from build123d import *

# Parameters (mm, degrees)
SKETCH_1_R      = 1.5
SKETCH_1_R_2    = 2
SKETCH_1_R_3    = 6.2
EXTRUDE_1_DEPTH = 3


with BuildPart() as part:
    # 草图1 → 凸台-拉伸1 (new body)
    with BuildSketch(Plane.XY):
        with BuildLine():
            Line((2522.174251857, 1992.03397428), (2522.174251857, 1983.327521496))
            Line((2522.174251857, 1983.327521496), (2519.174251857, 1983.327521496))
            Line((2519.174251857, 1983.327521496), (2519.174251857, 1975.827521496))
            Line((2519.174251857, 1975.827521496), (2522.174251857, 1975.827521496))
            Line((2522.174251857, 1975.827521496), (2522.174251857, 1965.121068713))
            Line((2522.174251857, 1965.121068713), (2517.424251857, 1965.121068713))
            Line((2517.424251857, 1965.121068713), (2517.424251857, 1968.121068713))
            Line((2517.424251857, 1968.121068713), (2509.924251857, 1968.121068713))
            Line((2509.924251857, 1968.121068713), (2509.924251857, 1965.121068713))
            Line((2509.924251857, 1965.121068713), (2498.924251857, 1965.121068713))
            Line((2498.924251857, 1965.121068713), (2498.924251857, 1968.121068713))
            Line((2498.924251857, 1968.121068713), (2491.424251857, 1968.121068713))
            Line((2491.424251857, 1968.121068713), (2491.424251857, 1965.121068713))
            Line((2491.424251857, 1965.121068713), (2480.424251857, 1965.121068713))
            Line((2480.424251857, 1965.121068713), (2480.424251857, 1968.121068713))
            Line((2480.424251857, 1968.121068713), (2472.924251857, 1968.121068713))
            Line((2472.924251857, 1968.121068713), (2472.924251857, 1965.121068713))
            Line((2472.924251857, 1965.121068713), (2468.174251857, 1965.121068713))
            Line((2468.174251857, 1965.121068713), (2468.174251857, 1975.827521496))
            Line((2468.174251857, 1975.827521496), (2471.174251857, 1975.827521496))
            Line((2471.174251857, 1975.827521496), (2471.174251857, 1983.327521496))
            Line((2471.174251857, 1983.327521496), (2468.174251857, 1983.327521496))
            Line((2468.174251857, 1983.327521496), (2468.174251857, 1992.03397428))
            ThreePointArc((2468.174251857, 1992.03397428), (2495.174251857, 2019.03397428), (2522.174251857, 1992.03397428))
        make_face()
        with Locations((2472.663889086, 1992.03397428)):
            Circle(SKETCH_1_R, mode=Mode.SUBTRACT)
        with Locations((2483.919070472, 2011.528520288)):
            Circle(SKETCH_1_R, mode=Mode.SUBTRACT)
        with Locations((2506.429433243, 2011.528520288)):
            Circle(SKETCH_1_R, mode=Mode.SUBTRACT)
        with Locations((2517.684614628, 1992.03397428)):
            Circle(SKETCH_1_R, mode=Mode.SUBTRACT)
        with Locations((2501.338054428, 1969.0074786)):
            Circle(SKETCH_1_R_2, mode=Mode.SUBTRACT)
        with Locations((2483.919070472, 1972.539428272)):
            Circle(SKETCH_1_R, mode=Mode.SUBTRACT)
        with Locations((2506.429433243, 1972.539428272)):
            Circle(SKETCH_1_R, mode=Mode.SUBTRACT)
        with Locations((2489.010449286, 1969.0074786)):
            Circle(SKETCH_1_R_2, mode=Mode.SUBTRACT)
        with Locations((2495.174251857, 1992.03397428)):
            Circle(SKETCH_1_R_3, mode=Mode.SUBTRACT)
    extrude(amount=EXTRUDE_1_DEPTH)


solid = part.part
Part model, mm, in its own coordinate system. A direction names the side the tool comes from. Give positions to 0.01 mm unless a question says otherwise; leave off trailing zeros. Write each loop counter-clockwise with the first axis right and the second up, starting at its lowest first coordinate (ties: lowest second). Pieces come first, ordered by that corner, then holes.
1) Two-plate mould, pull along Y, no slides. Class faces 1 (the face through (2486, 1965.121, 1)), 2 (the face through (2500.9, 1989.66, 1.48)), 3 (the face through (2509.924, 1967, 1)): released by +Y, released by -Y, zero draft, split by the parting line, or undercut.
Resolved:
face 1: released by -Y
face 2: undercut
face 3: zero draft
2) Cut at A-A on y = 1989.5. Write the cut outline in (x, z).
Resolved:
outline: (2468.17, 0) - (2489.52, 0) - (2489.52, 3) - (2468.17, 3) - close; (2500.83, 0) - (2522.17, 0) - (2522.17, 3) - (2500.83, 3) - close
3) Cut at B-B on x = 2497. Write the cut outline in (y, z).
Resolved:
outline: (1968.12, 0) - (1986.11, 0) - (1986.11, 3) - (1968.12, 3) - close; (1997.96, 0) - (2018.97, 0) - (2018.97, 3) - (1997.96, 3) - close
4) Which spindle directions (+Z, -Z, +X, -X, +Y, -Y) get a long thin tool onto all of the face, cutting with end or side? Do faces 4 (the face through (2505, 1973, 1)), 5 (the face through (2495, 1968.121, 1)), 6 (the face through (2521, 1983.328, 1)), 7 (the face through (2471.174, 1980, 1)), 8 (the face through (2502, 1992, 3)). Say none if no direction does.
Resolved:
face 4: +Z, -Z
face 5: +Z, -Z, -Y
face 6: +Z, -Z, +X
face 7: +Z, -Z, -X
face 8: +Z, +X, -X, +Y, -Y
5) Cut at C-C on z = 2. State how many separate pieces and enclosed holes the cut face has, then the cut area to 3 significant figures.
Resolved:
separate pieces: 1
enclosed holes: 9
area: 2,300 mm2
6) Cut at D-D on y = 1978. Write the cut outline in (x, z).
Resolved:
outline: (2471.17, 0) - (2519.17, 0) - (2519.17, 3) - (2471.17, 3) - close
7) Probe L1, parallel to X at y = 1969, z = 2.3; L2, parallel to X at y = 1972.5, z = 0.65; L3, parallel to X at y = 1992.5, z = 2.7. List the from-to ranges inside material, lowest first.
Resolved:
L1: x = 2468.17 to 2487.01, 2491.01 to 2499.34, 2503.34 to 2522.17
L2: x = 2468.17 to 2482.42, 2485.42 to 2504.93, 2507.93 to 2522.17
L3: x = 2468.18 to 2471.24, 2474.09 to 2488.99, 2501.36 to 2516.26, 2519.11 to 2522.17
8) Pin check, flat tips, straight feed: pin 1 (1.5 mm diameter, centred on y = 1999.5, z = 0.5, fed in from +X); pin 2 (2.5 mm diameter, centred on x = 2483.92, y = 2011.53, fed in from +Z); pin 3 (0.9 mm diameter, centred on y = 1980, z = 1.5, fed in from +X). Stop position of each tip, or through.
Resolved:
pin 1: stops at x = 2521.33
pin 2: passes through
pin 3: stops at x = 2519.17
